Can you work these out from the drawing? Everything is in mm from the part's minimum corner. A direction names the side the tool comes from. Round coordinates to 2 decimals unless told otherwise and drop trailing zeros. Write each loop counter-clockwise with the first axis right and the second up, starting at its lowest first coordinate (ties: lowest second). Pieces come first, ordered by that corner, then holes. Notation, with made-up numbers: (33, 49) -> (52, 49) arc R17 cw to (52, 74) -> close; hole circle Ø3 at (85, 14.5). An arc over 180 degrees is marked (long way). Write item = value, one per line. Start each with the question number.
1) Imagine slicing it at C-C, the plane z = 3.5. Please give me the cut outline in (x, y) (1 decimal).
2) Imagine slicing it at A-A, the plane z = 6.35. Please give me the cut outline in (x, y) (1 decimal).
3) If I drill on line 1 (Z direction, x = 34, y = 4.25); line 2 (Y direction, x = 21, z = 8); line 3 (X direction, y = 15, z = 9) (1 decimal), over which ranges is the centre line in solid material (lowest first)?
4) For the marked faces 1, 2 and 3, which set-ups out of +Z, -Z, +X, -X, +Y, -Y let a thin tool reach every point of the face, with its end or its side?
5) I'm going to push flat-ended pins straight in: pin 1 (1.5 mm diameter, centred on y = 16, z = 7.5, fed in from +X); pin 2 (2 mm diameter, centred on x = 21.5, z = 1.5, fed in from -Y); pin 3 (6 mm diameter, centred on x = 33.5, z = 3.5, fed in from +Y) (1 decimal); pin 4 (5 mm diameter, centred on x = 20.92, y = 22.5, fed in from -Z). Where does each tip first touch, or does it pass through?
6) Imagine slicing it at D-D, the plane x = 34.5. Please give me the cut outline in (y, z) (1 decimal).
7) Imagine slicing it at B-B, the plane y = 22.5. Please give me the cut outline in (x, z) (1 decimal).
8) Thinking about a two-plate mould opening in Z: for the marked faces 4, 5, 6 and 7, which applies, +Z half, -Z half, draft (parallel to the pull), parting line (faces both ways), or undercut?
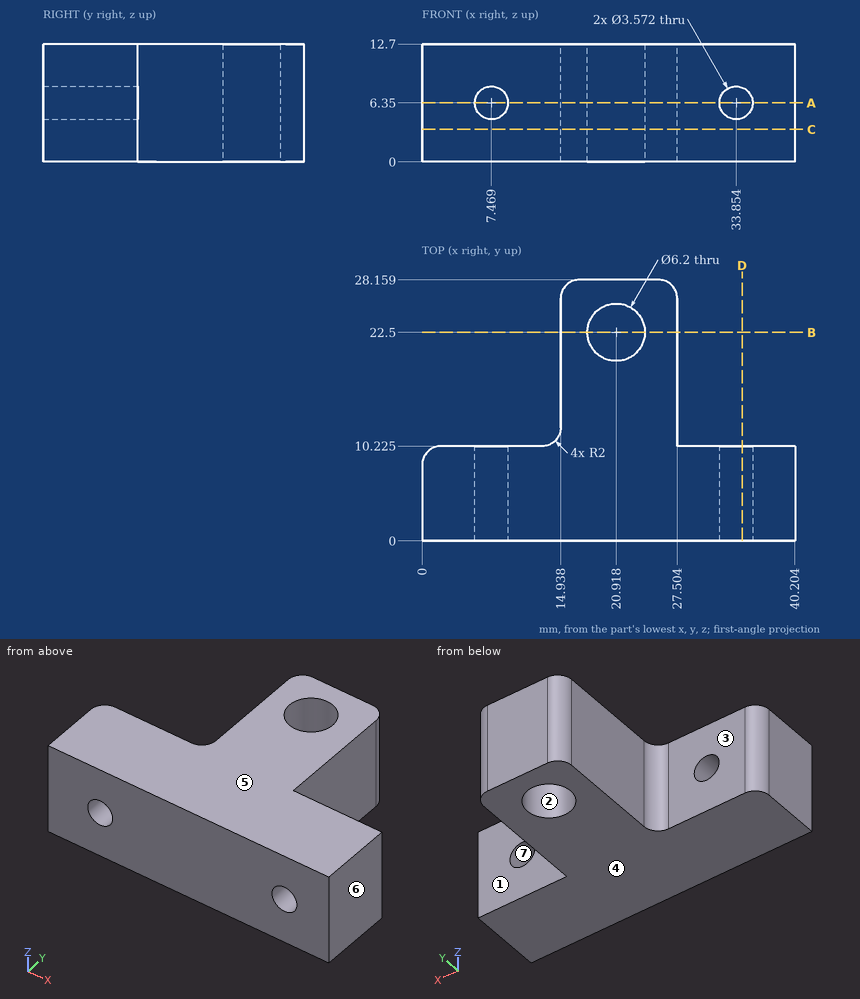
Reported:
q1.outline = (0, 0) -> (40.2, 0) -> (40.2, 10.2) -> (27.5, 10.2) -> (27.5, 26.2) arc R2 ccw to (25.5, 28.2) -> (16.9, 28.2) arc R2 ccw to (14.9, 26.2) -> (14.9, 12.2) arc R2 cw to (12.9, 10.2) -> (2, 10.2) arc R2 ccw to (0, 8.2) -> close; hole circle Ø6.2 at (20.9, 22.5)
q2.outline = (0, 0) -> (5.7, 0) -> (5.7, 10.2) -> (2, 10.2) arc R2 ccw to (0, 8.2) -> close; (9.3, 0) -> (32.1, 0) -> (32.1, 10.2) -> (27.5, 10.2) -> (27.5, 26.2) arc R2 ccw to (25.5, 28.2) -> (16.9, 28.2) arc R2 ccw to (14.9, 26.2) -> (14.9, 12.2) arc R2 cw to (12.9, 10.2) -> (9.3, 10.2) -> close; (35.6, 0) -> (40.2, 0) -> (40.2, 10.2) -> (35.6, 10.2) -> close; hole circle Ø6.2 at (20.9, 22.5)
q3.line_1 = 0 to 4.57, 8.13 to 12.7
q3.line_2 = 0 to 19.4, 25.6 to 28.16
q3.line_3 = 14.9 to 27.5
q4.face_1 = +Z, -Z, +X, +Y
q4.face_2 = +Z, -Z
q4.face_3 = +Z, -Z, -X, +Y
q5.pin_1 = 27.5
q5.pin_2 = 0
q5.pin_3 = 10.2
q5.pin_4 = through
q6.outline = (0, 0) -> (10.2, 0) -> (10.2, 4.7) -> (0, 4.7) -> close; (0, 8) -> (10.2, 8) -> (10.2, 12.7) -> (0, 12.7) -> close
q7.outline = (14.9, 0) -> (17.8, 0) -> (17.8, 12.7) -> (14.9, 12.7) -> close; (24, 0) -> (27.5, 0) -> (27.5, 12.7) -> (24, 12.7) -> close
q8.face_4 = -Z half
q8.face_5 = +Z half
q8.face_6 = draft
q8.face_7 = undercut
